Geometry check sheet. Reference: the model listing, model coordinates, mm. A direction names the side the tool comes from. Round coordinates to 2 decimals unless told otherwise and drop trailing zeros. Loops run counter-clockwise (first coordinate to the right, second up) from the corner with the lowest first, then second, coordinate; pieces in that order, holes last. Notation, with made-up numbers: (74, 79.25) -> (89, 79.25) arc R18 ccw to (89, 113.25) -> close; hole circle Ø1 at (19.25, 35). An arc over 180 degrees is marked (long way). Use a Markdown table: item, result. Add a question column.
Q1. Gauge pin test, flat ends, axial feed: P1, Ø6.5, axis at x = 32.5, y = 0.5, coming from the -Z side; P2, Ø3, axis at y = 6, z = -3.5, coming from the -X side; P3, Ø1.5, axis at y = 3.5, z = -5.5, coming from the +X side. Record the tip position at first contact, or that the pin passes through.
Q2. Sectioned sample at A-A, the plane z = -3. Give the number of separate pieces and of enclosed holes in the cut face, then the cut area to 3 significant figures.
Q3. Material ranges on L1, parallel to X at y = -4.5, z = -2.5; L2, parallel to X at y = -29, z = -3; L3, parallel to Y at x = 34, z = -5, recorded low to high.
Q4. Release check for a two-part mould opening along Y. For faces 1 (the face through (22, 0, -6.35)), 2 (the face through (-10.19, 45.87, -2.82)), 3 (the face through (-19.05, 1, -3)), 4 (the face through (26.397, -21.455, -3.219)) record: released by +Y, released by -Y, zero draft, split by the parting line, or undercut.
Q5. Set-up check for faces 5 (the face through (20, 1, 0)), 6 (the face through (-0.277, -41.274, -3.131)), 7 (the face through (31, -5, -1.575)): record each of +Z, -Z, +X, -X, +Y, -Y from which the full face is reachable in a straight line by a thin tool's end or side.
Q6. Sectioned sample at B-B, the plane x = 0. Enter the section's corners in (y, z) (3 decimals).
Autodesk Inventor part; units mm, degrees
ref_plane "YZ Plane" through (0, 0, 0) normal (1, 0, 0) x (0, 1, 0)
ref_plane "XZ Plane" through (0, 0, 0) normal (0, 1, 0) x (-1, 0, 0)
ref_plane "XY Plane" through (0, 0, 0) normal (0, 0, 1) x (1, 0, 0)
sketch "Sketch1" plane through (0, 0, 0) normal (0, 1, 0) x (-1, 0, 0)
  line L0 (0, 0) -> (-46.99, 0)
  line L1 (-46.99, 0) -> (-46.99, -5.5563)
  line L2 (-46.99, -5.5563) -> (0, -5.5562)
  line L3 (0, -5.5562) -> (0, 0)
  line L4 (-44.45, -4.1049) -> (-42.2049, -6.35)
  line L5 (-42.2049, -6.35) -> (-44.45, -8.5951)
  line L6 (-44.45, -8.5951) -> (-46.6951, -6.35)
  line L7 (-46.6951, -6.35) -> (-44.45, -4.1049)
  line L8 (-42.2049, -6.35) -> (0, -6.35)
  line L9 (0, -6.35) -> (0, -5.5562)
  point P0 (-44.45, -6.35)
  point P1 (-45.9013, -5.5563)
  dimension "d0" = 46.99
  dimension "d2" = 3.175
  dimension "d3" = 6.35
  dimension "d4" = 44.45
  dimension "d10" = 0.7937
revolve "Revolution1" add sketch "Sketch1" angle 360 about axis through (0, 0, -5.5562) along (0, 0, 1) contours L3 L2 L4 L7 L1 L0 | L9 L8 L4 L2
sketch "Sketch2" plane through (0, 0, 0) normal (0, 0, 1) x (1, 0, 0)
  circle A0 centre (0, 0) radius 41.275
  line L0 (-19.05, 36.6159) -> (-19.05, -36.6159)
  line L1 (19.05, -36.6159) -> (19.05, 36.6159)
  point P0 (0, 0)
  dimension "d6" = 82.55
  dimension "d7" = 38.1
extrude "Extrusion1" cut sketch "Sketch2" against normal through all contours L1 A0 L0
sketch "Sketch3" plane through (0, 0, 0) normal (0, 0, 1) x (1, 0, 0)
  line L0 (25.4, -19.05) -> (-25.4, -19.05) construction
  line L1 (-25.4, -19.05) -> (-25.4, 19.05) construction
  line L2 (-25.4, 19.05) -> (25.4, 19.05) construction
  line L3 (25.4, 19.05) -> (25.4, -19.05) construction
  line L4 (25.4, -19.05) -> (-25.4, 19.05) construction
  line L5 (25.4, 19.05) -> (-25.4, -19.05) construction
  point P0 (0, 0)
  point P1 (0, 0)
  dimension "d11" = 50.8
  dimension "d12" = 38.1
hole "Hole1" at (25.4, -19.05, 0) at (25.4, 19.05, 0) at (-25.4, 19.05, 0) at (-25.4, -19.05, 0) direction (0, 0, -1) diameter 5.207 end through all
sketch "Sketch4" plane through (0, 0, -6.35) normal (0, 0, -1) x (-1, 0, 0)
  circle A0 centre (0, 0) radius 30.48 construction
  point P0 (0, 0)
  point P1 (-30.48, 0)
  point P2 (30.48, 0)
  dimension "d20" = 60.96
hole "Hole2" at (30.48, 0, -6.35) at (-30.48, 0, -6.35) direction (0, 0, 1) diameter 9.525 end through all counterbore diameter 12.954 counterbore depth 4.7752
properties part number "CarriageCap_V4" material "ABS Plastic"
Values:
| question | item | result |
|---|---|---|
| 1 | P1 | z = -1.57 |
| 1 | P2 | x = -46.77 |
| 1 | P3 | x = 46.91 |
| 2 | separate pieces | 1 |
| 2 | enclosed holes | 7 |
| 2 | area | 3,560 mm^2 |
| 3 | L1 | -46.77 to -35.14, -25.82 to -19.05, 19.05 to 25.82, 35.14 to 46.77 |
| 3 | L2 | -36.97 to -19.05, 19.05 to 36.97 |
| 3 | L3 | -32.44 to -30, -27.22 to -5.44, 5.44 to 27.22, 30 to 32.44 |
| 4 | face 1 | zero draft |
| 4 | face 2 | split by the parting line |
| 4 | face 3 | undercut |
| 4 | face 4 | undercut |
| 5 | face 5 | +Z, +X, -X, +Y, -Y |
| 5 | face 6 | +Z, -Z |
| 5 | face 7 | -Z |
| 6 | outline | (-46.99, -5.556) -> (-45.901, -5.556) -> (-44.45, -4.105) -> (-42.205, -6.35) -> (-41.275, -6.35) -> (-41.275, 0) -> (-46.99, 0) -> close; (41.275, -6.35) -> (42.205, -6.35) -> (44.45, -4.105) -> (45.901, -5.556) -> (46.99, -5.556) -> (46.99, 0) -> (41.275, 0) -> close |
